Part print with two shaded views. Sizes in mm from the minimum x, y, z corner. Coordinates: 2 decimals unless noted, no trailing zeros. Loops run counter-clockwise (first coordinate to the right, second up) from the corner with the lowest first, then second, coordinate; pieces in that order, holes last.
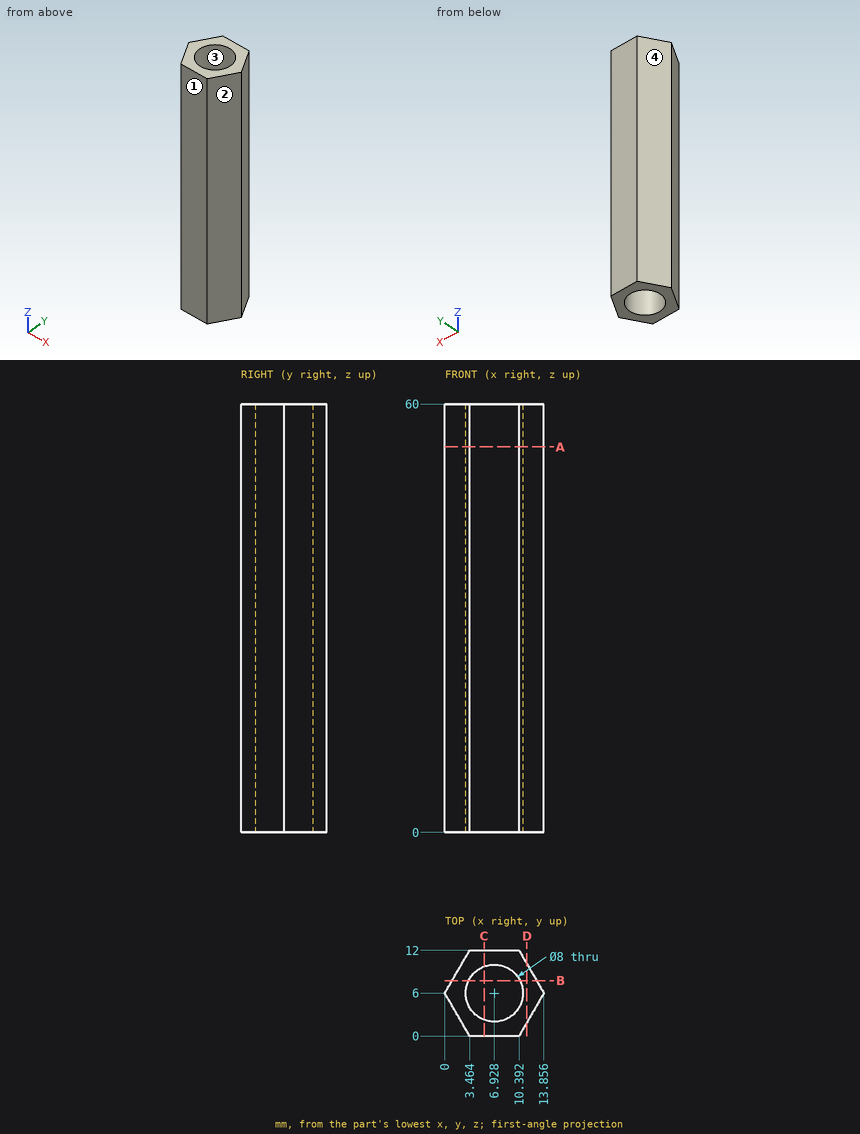
Q1. Slice it at B-B (y = 7.75). List the corners of the cut face in (x, z) (1 decimal).
Answers:
outline: (1, 0) - (3.3, 0) - (3.3, 60) - (1, 60) - close; (10.5, 0) - (12.8, 0) - (12.8, 60) - (10.5, 60) - close
Q2. Slice it at D-D (x = 11.5). List the corners of the cut face in (y, z), and give its area (3 significant figures).
Answers:
outline: (1.92, 0) - (10.08, 0) - (10.08, 60) - (1.92, 60) - close
area: 490 mm2
Q3. Slice it at C-C (x = 5.5). List the corners of the cut face in (y, z).
Answers:
outline: (0, 0) - (2.26, 0) - (2.26, 60) - (0, 60) - close; (9.74, 0) - (12, 0) - (12, 60) - (9.74, 60) - close
Q4. Slice it at A-A (z = 54). List the corners of the cut face in (x, y).
Answers:
outline: (0, 6) - (3.46, 0) - (10.39, 0) - (13.86, 6) - (10.39, 12) - (3.46, 12) - close; hole circle Ø8 at (6.93, 6)
Q5. Flat gauge pin, fed straight in: P1, Ø2, axis at y = 6.5, z = 39, coming from the -X side. Where does the tip first touch, or does it go through?
Answers:
P1: stops at x = 0
Q6. Mould opens along X. For the marked faces 1, 2, 3 and 4 say: +X half, -X half, draft (parallel to the pull), parting line (faces both ways), or undercut.
Answers:
face 1: draft
face 2: +X half
face 3: undercut
face 4: -X half
Q7. Drill centre lines: line 1 (Y direction, x = 7, z = 5); line 2 (Y direction, x = 8.25, z = 39) (1 decimal); line 3 (X direction, y = 5.5, z = 50.5). Where is each one in solid material? Low to high.
Answers:
line 1: y = 0 to 2, 10 to 12
line 2: y = 0 to 2.2, 9.8 to 12
line 3: x = 0.29 to 2.96, 10.9 to 13.57
